Solid Edge part; units mm, degrees
sketch "Sketch1" plane through (0, 0, 0) normal (0, -1, 0) x (1, 0, 0)
  circle A0 centre (-38, 73) radius 1.7
  circle A1 centre (-22.2, 73) radius 1.7
  circle A2 centre (-22.2, 47) radius 1.7
  circle A3 centre (-38, 47) radius 1.7
  line L0 (-42, 79) -> (-42, 41)
  line L1 (-19, 41) -> (-42, 41)
  line L2 (-19, 51.3832) -> (-19, 41)
  line L3 (-19, 79) -> (-19, 68.6168)
  line L4 (-19, 79) -> (-42, 79)
  arc A4 (-19, 51.3832) -> (-19, 68.6168) centre (-15, 60) cw
extrude "Protrusion1" add sketch "Sketch1" along normal blind 9
sketch "Sketch2" plane through (-29.9, -4, 41) normal (0, 0, -1) x (0, -1, 0)
  circle A0 centre (-4, 0.1) radius 4.2
extrude "Cutout1" cut sketch "Sketch2" against normal through all
sketch "Sketch3" plane through (-29.9, -4, 66.2) normal (0, 0, 1) x (0, -1, 0)
  circle A0 centre (-4, -0.1) radius 6.2
extrude "ExtrudedCutout_2" cut sketch "Sketch3" against normal blind 1.5
sketch "Sketch4" plane through (-29.9, -9, 61.3992) normal (0, -1, 0) x (-1, 0, 0)
  circle A0 centre (8.1, 1.3992) radius 1.7
extrude "Cutout2" cut sketch "Sketch4" against normal through all
Verification items for the finished model (mm, model axes). A direction names the side the tool comes from. Coordinates: 2 decimals unless noted, no trailing zeros. Write each loop counter-clockwise with the first axis right and the second up, starting at its lowest first coordinate (ties: lowest second). Pieces come first, ordered by that corner, then holes. Notation, with made-up numbers: (-31, 52) -> (-10, 52) arc R8 ccw to (-10, 57) -> close; hole circle Ø7 at (10.25, -6). An arc over 180 degrees is marked (long way). One line per item, written item: value. Start each with the question number.
Q1. Cross-section at D-D on z = 73. Enter the section's corners in (x, y), and give its area (3 significant figures).
Q2. Thickness scan on L1, parallel to Z at x = -38, y = -5.75; L2, parallel to Z at x = -23.5, y = -7.5; L3, parallel to Z at x = -35.75, y = -1. Record the ranges inside material, lowest first. Write a range as from..to.
Q3. Cross-section at B-B on y = -2.5. Enter the section's corners in (x, z).
Q4. Access from +Z, -Z, +X, -X, +Y, -Y to the whole of each face (thin tool, end or side, straight path). Record for faces 4 (the cylindrical face through (-30.1, -6.2, 65.5)), 5 (the cylindrical face through (-23.55, -4.44, 48.03)).
Q5. Cross-section at C-C on x = -38. Enter the section's corners in (y, z).
Q6. Cross-section at A-A on z = 60. Enter the section's corners in (x, y).
Q7. Mould release check, pull along Z, two halves, no side actions. Record for faces 1 (the flat face through (-30.3, -4.4, 41)), 2 (the flat face through (-25, 0, 60)), 3 (the flat face through (-30.1, -4.4, 66.2)): pulls with the +Z half, pulls with the -Z half, needs draft (parallel to the pull), parting line crosses it, or undercut.
Q8. Go/stop test with a flat-tipped pin: P1, Ø1.9, axis at x = -31.5, y = -2.5, coming from the -Z side. Record where the tip stops, or that it passes through.
Checked values:
1. outline: (-42, -9) -> (-39.7, -9) -> (-39.7, 0) -> (-42, 0) -> close; (-36.3, -9) -> (-23.9, -9) -> (-23.9, 0) -> (-25.8, 0) arc R4.2 cw to (-34.2, 0) -> (-36.3, 0) -> close; (-20.5, -9) -> (-19, -9) -> (-19, 0) -> (-20.5, 0) -> close
1. area: 118 mm²
2. L1: z = 41..45.3, 48.7..58.3, 61.7..71.3, 74.7..79
2. L2: z = 41..45.9, 48.1..55.76, 64.24..71.9, 74.1..79
2. L3: z = 41..64.7, 66.2..79
3. outline: (-42, 41) -> (-33.37, 41) -> (-33.37, 64.7) -> (-35.67, 64.7) -> (-35.67, 66.2) -> (-33.37, 66.2) -> (-33.37, 79) -> (-42, 79) -> close; (-26.63, 41) -> (-19, 41) -> (-19, 51.38) arc R9.5 cw to (-19, 68.62) -> (-19, 79) -> (-26.63, 79) -> (-26.63, 66.2) -> (-24.33, 66.2) -> (-24.33, 64.7) -> (-26.63, 64.7) -> close; hole circle Ø3.4 at (-38, 47); hole circle Ø3.4 at (-38, 60); hole circle Ø3.4 at (-38, 73); hole circle Ø3.4 at (-22.2, 47); hole circle Ø3.4 at (-22.2, 73)
4. face 4: +Y
4. face 5: +Y, -Y
5. outline: (-9, 41) -> (0, 41) -> (0, 45.3) -> (-9, 45.3) -> close; (-9, 48.7) -> (0, 48.7) -> (0, 58.3) -> (-9, 58.3) -> close; (-9, 61.7) -> (0, 61.7) -> (0, 71.3) -> (-9, 71.3) -> close; (-9, 74.7) -> (0, 74.7) -> (0, 79) -> (-9, 79) -> close
6. outline: (-42, -9) -> (-39.7, -9) -> (-39.7, 0) -> (-42, 0) -> close; (-36.3, -9) -> (-24.5, -9) -> (-24.5, 0) -> (-25.8, 0) arc R4.2 cw to (-34.2, 0) -> (-36.3, 0) -> close
7. face 1: pulls with the -Z half
7. face 2: needs draft
7. face 3: undercut
8. P1: passes through
